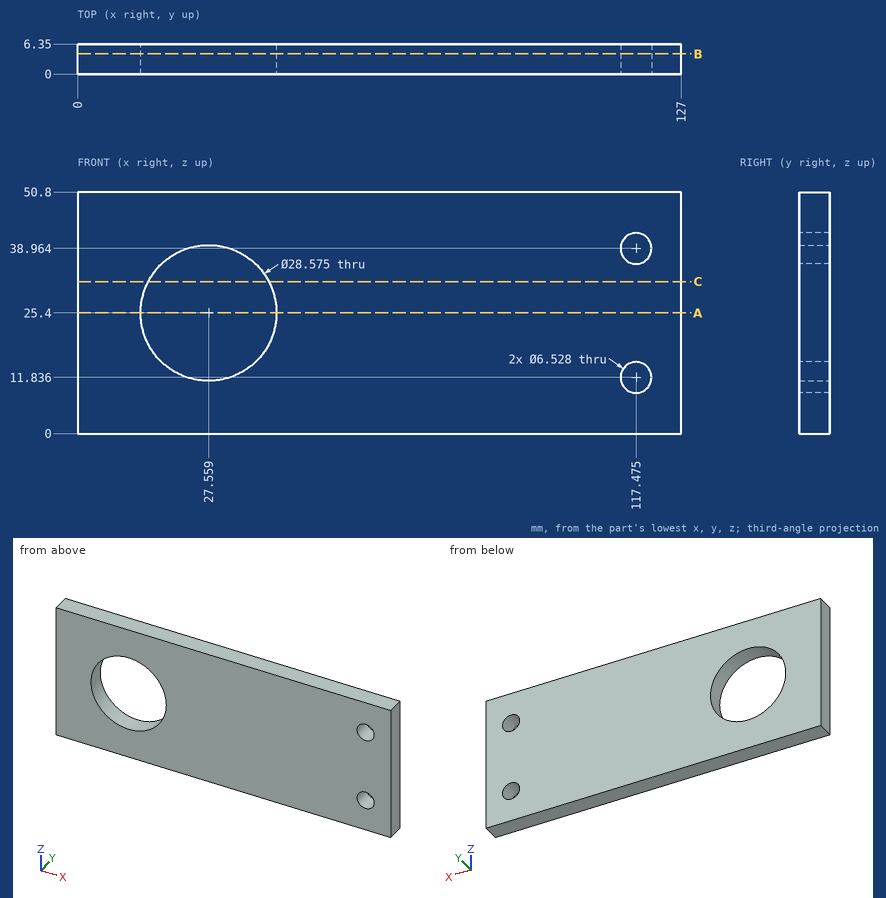
Print and shaded views of the part. All mm, measured from the part's lowest x, y and z. Coordinates: 2 decimals unless noted, no trailing zeros. Order: outer loops, then holes, each group sorted by start corner. A loop starts at its lowest first (then second) coordinate and runs counter-clockwise, first axis right, second up.
Item 1: Drill centre lines: L1, parallel to X at y = 2, z = 25.4; L2, parallel to Z at x = 37.5, y = 1.75; L3, parallel to Z at x = 34, y = 1.5. Where is each one in solid material? Low to high.
Filled in:
L1: x = 0 to 13.27, 41.85 to 127
L2: z = 0 to 15.14, 35.66 to 50.8
L3: z = 0 to 12.65, 38.15 to 50.8
Item 2: Saw through at A-A on z = 25.4. List the corners of the cut face in (x, y), then the cut area to 3 significant figures.
Filled in:
outline: (0, 0) - (13.27, 0) - (13.27, 6.35) - (0, 6.35) - close; (41.85, 0) - (127, 0) - (127, 6.35) - (41.85, 6.35) - close
area: 625 mm2
Item 3: Drop a flat-ended pin along its axis: pin 1 Ø1 at (x, z) = (36.5, 37) entering from -Y. Give the stop position or say it passes through.
Filled in:
pin 1: stops at y = 0
Item 4: Saw through at C-C on z = 32. List the corners of the cut face in (x, y).
Filled in:
outline: (0, 0) - (14.89, 0) - (14.89, 6.35) - (0, 6.35) - close; (40.23, 0) - (127, 0) - (127, 6.35) - (40.23, 6.35) - close
Item 5: Saw through at B-B on y = 4.25. List the corners of the cut face in (x, z) (1 decimal), then the cut area to 3 significant figures.
Filled in:
outline: (0, 0) - (127, 0) - (127, 50.8) - (0, 50.8) - close; hole circle Ø28.6 at (27.6, 25.4); hole circle Ø6.5 at (117.5, 11.8); hole circle Ø6.5 at (117.5, 39)
area: 5,740 mm2
